from build123d import *

# Parameters (mm, degrees)
AUFSATZ_LINEAR_AUSTRAGEN1_DEPTH  = 13
AUFSATZ_LINEAR_START             = -13
SKIZZE2_W                        = 3
SKIZZE2_H                        = 12
AUFSATZ_LINEAR_AUSTRAGEN2_DEPTH  = 45
SKIZZE3_W                        = 8.8
SKIZZE3_H                        = 13
SKIZZE3_W_2                      = 18.8
AUFSATZ_LINEAR_AUSTRAGEN3_DEPTH  = 16.6
SKIZZE4_R                        = 1.7
SCHNITT_LINEAR_AUSTRAGEN1_DEPTH  = 4
SKIZZE6_R                        = 1.5
SCHNITT_LINEAR_AUSTRAGEN2_DEPTH  = 4
SCHNITT_LINEAR_START             = -3
SCHNITT_LINEAR_AUSTRAGEN4_DEPTH  = 2.5
SCHNITT_LINEAR_AUSTRAGEN6_DEPTH  = 91
SCHNITT_LINEAR_AUSTRAGEN7_REACH  = 2.5
SKIZZE11_R                       = 3.85
SCHNITT_LINEAR_START_2           = -15
SKIZZE12_W                       = 8
SKIZZE12_H                       = 5
SCHNITT_LINEAR_AUSTRAGEN8_DEPTH  = 16
SKIZZE13_W                       = 5
SKIZZE13_H                       = 8
SCHNITT_LINEAR_AUSTRAGEN9_DEPTH  = 91
SKIZZE14_R                       = 1
SCHNITT_LINEAR_AUSTRAGEN10_DEPTH = 71
AUFSATZ_LINEAR_START_2           = -3
SKIZZE15_R                       = 6
AUFSATZ_LINEAR_AUSTRAGEN4_DEPTH  = 4
SKIZZE16_R                       = 1.7
SCHNITT_LINEAR_AUSTRAGEN11_DEPTH = 3


with BuildPart() as part:
    # Skizze1 → Aufsatz-Linear austragen1 (new body)
    with BuildSketch(Plane.XY):
        Polygon((-45, 67), (-42, 67), (-42, 0), (42, 0), (42, 67), (45, 67), (45, -3), (-45, -3), align=None)
    extrude(amount=AUFSATZ_LINEAR_AUSTRAGEN1_DEPTH)

    # Skizze2 → Aufsatz-Linear austragen2 (add)
    with BuildSketch(Plane(origin=(0, 0, 0), x_dir=(-1, 0, 0), z_dir=(0, 0, -1)).offset(AUFSATZ_LINEAR_START)):
        with Locations((-43.5, 61)):
            Rectangle(SKIZZE2_W, SKIZZE2_H)
        with Locations((43.5, 61)):
            Rectangle(SKIZZE2_W, SKIZZE2_H)
    extrude(amount=AUFSATZ_LINEAR_AUSTRAGEN2_DEPTH)

    # Skizze3 → Aufsatz-Linear austragen3 (add)
    with BuildSketch(Plane(origin=(0, 0, 0), x_dir=(1, 0, 0), z_dir=(0, 1, 0))):
        with Locations((-37.6, -6.5)):
            Rectangle(SKIZZE3_W, SKIZZE3_H)
        with Locations((37.6, -6.5)):
            Rectangle(SKIZZE3_W, SKIZZE3_H)
        with Locations((0, -6.5)):
            Rectangle(SKIZZE3_W_2, SKIZZE3_H)
    extrude(amount=AUFSATZ_LINEAR_AUSTRAGEN3_DEPTH)

    # Skizze4 → Schnitt-Linear austragen1 (cut)
    with BuildSketch(Plane(origin=(0, 16.6, 0), x_dir=(1, 0, 0), z_dir=(0, 1, 0))):
        with Locations((-35.6, -6.5)):
            Circle(SKIZZE4_R)
        with Locations((-7, -6.5)):
            Circle(SKIZZE4_R)
        with Locations((7, -6.5)):
            Circle(SKIZZE4_R)
        with Locations((35.6, -6.5)):
            Circle(SKIZZE4_R)
    extrude(amount=-SCHNITT_LINEAR_AUSTRAGEN1_DEPTH, mode=Mode.SUBTRACT)

    # Skizze6 → Schnitt-Linear austragen2 (cut, through all)
    with BuildSketch(Plane.ZY.offset(-42)):
        with Locations((-26, 61)):
            Circle(SKIZZE6_R)
    extrude(amount=-SCHNITT_LINEAR_AUSTRAGEN2_DEPTH, mode=Mode.SUBTRACT)

    # Skizze7 → Schnitt-Linear austragen4 (cut)
    with BuildSketch(Plane.ZY.offset(45).offset(SCHNITT_LINEAR_START)):
        with BuildLine():
            Line((-25.802102804, 64.844910493), (-4.45864486, 63.746364638))
            ThreePointArc((-4.45864486, 63.746364638), (-1.85, 61), (-4.45864486, 58.253635362))
            Line((-4.45864486, 58.253635362), (-25.802102804, 57.155089507))
            ThreePointArc((-25.802102804, 57.155089507), (-29.85, 61), (-25.802102804, 64.844910493))
        make_face()
    extrude(amount=SCHNITT_LINEAR_AUSTRAGEN4_DEPTH, mode=Mode.SUBTRACT)

    # Skizze10 → Schnitt-Linear austragen6 (cut, through all)
    with BuildSketch(Plane.ZY.offset(45)):
        with BuildLine():
            Line((-26, 55), (-40.113250667, 55))
            Line((-40.113250667, 55), (-40.113250667, 67))
            Line((-40.113250667, 67), (-26, 67))
            ThreePointArc((-26, 67), (-32, 61), (-26, 55))
        make_face()
    extrude(amount=-SCHNITT_LINEAR_AUSTRAGEN6_DEPTH, mode=Mode.SUBTRACT)

    # Skizze11 → Schnitt-Linear austragen7 (cut, up to next)
    with BuildSketch(Plane(origin=(-44.5, 0, 0), x_dir=(0, 0, -1), z_dir=(1, 0, 0)), mode=Mode.PRIVATE) as schnitt_linear_austragen7_sk1:
        with Locations((26, 61)):
            Circle(SKIZZE11_R)
    schnitt_linear_austragen7_tool1 = extrude(schnitt_linear_austragen7_sk1.sketch, amount=-SCHNITT_LINEAR_AUSTRAGEN7_REACH, mode=Mode.PRIVATE) & part.part
    add(schnitt_linear_austragen7_tool1.solids().sort_by_distance((-44.5, 61, -26))[0], mode=Mode.SUBTRACT)

    # Skizze12 → Schnitt-Linear austragen8 (cut)
    with BuildSketch(Plane(origin=(45, 0, 0), x_dir=(0, 0, -1), z_dir=(1, 0, 0)).offset(SCHNITT_LINEAR_START_2)):
        with Locations((-4, 3.5)):
            Rectangle(SKIZZE12_W, SKIZZE12_H)
    schnitt_linear_austragen8 = extrude(amount=SCHNITT_LINEAR_AUSTRAGEN8_DEPTH, mode=Mode.SUBTRACT)

    # Spiegeln1: Schnitt-Linear austragen8 across plane
    add(schnitt_linear_austragen8.mirror(Plane.ZY), mode=Mode.SUBTRACT)

    # Skizze13 → Schnitt-Linear austragen9 (cut, through all)
    with BuildSketch(Plane.ZY.offset(45)):
        with Locations((6.5, 40.6)):
            Rectangle(SKIZZE13_W, SKIZZE13_H)
    extrude(amount=-SCHNITT_LINEAR_AUSTRAGEN9_DEPTH, mode=Mode.SUBTRACT)

    # Skizze14 → Schnitt-Linear austragen10 (cut, through all)
    with BuildSketch(Plane(origin=(0, -3, 0), x_dir=(-1, 0, 0), z_dir=(0, -1, 0))):
        with Locations((26.45, -6.15)):
            Circle(SKIZZE14_R)
        with Locations((-26.45, -6.15)):
            Circle(SKIZZE14_R)
    extrude(amount=-SCHNITT_LINEAR_AUSTRAGEN10_DEPTH, mode=Mode.SUBTRACT)

    # Skizze15 → Aufsatz-Linear austragen4 (add)
    with BuildSketch(Plane.ZY.offset(-42).offset(AUFSATZ_LINEAR_START_2)):
        with Locations((-26, 61)):
            Circle(SKIZZE15_R)
    extrude(amount=AUFSATZ_LINEAR_AUSTRAGEN4_DEPTH)

    # Skizze16 → Schnitt-Linear austragen11 (cut)
    with BuildSketch(Plane(origin=(45, 0, 0), x_dir=(0, 0, -1), z_dir=(1, 0, 0))):
        with Locations((26, 61)):
            Circle(SKIZZE16_R)
    extrude(amount=-SCHNITT_LINEAR_AUSTRAGEN11_DEPTH, mode=Mode.SUBTRACT)


solid = part.part
The listing builds one solid part. Answer for the finished solid, in the listing's coordinates (mm). A direction names the side the tool comes from. Coordinates: 2 decimals unless noted, no trailing zeros. Write each loop counter-clockwise with the first axis right and the second up, starting at its lowest first coordinate (ties: lowest second). Pieces come first, ordered by that corner, then holes. Notation, with made-up numbers: (-9.5, 78.5) - (-5.5, 78.5) arc R25 cw to (-5.5, 103.5) - close; hole circle Ø3 at (75.25, -17). An arc over 180 degrees is marked (long way). Put each result on its own line as item: value.
1. Determine the mould class of faces 4 (the face through (-9.4, 8, 7)), 5 (the face through (-43.48, 59.64, -29.6)), 6 (the face through (39, 3, 8)), 7 (the face through (43, 41, 9)) for opening direction Z: pulls with the +Z half, pulls with the -Z half, needs draft (parallel to the pull), parting line crosses it, or undercut.
Answer sheet:
face 4: needs draft
face 5: undercut
face 6: pulls with the -Z half
face 7: undercut
2. The part is cut by section A-A on y = 48.5. Give the vertices of the cut face in (x, z), plus the area to 3 significant figures.
Answer sheet:
outline: (-45, 0) - (-42, 0) - (-42, 13) - (-45, 13) - close; (42, 0) - (45, 0) - (45, 13) - (42, 13) - close
area: 78.0 mm^2
3. Flat-ended cylindrical pins translate along their axes: pin 1 Ø9.5 at (x, z) = (38, 4) entering from +Y; pin 2 Ø2.5 at (x, z) = (7, 7) entering from +Y; pin 3 Ø3 at (x, z) = (-7, 6.5) entering from +Y. Find the tip coordinate at first contact, or state that the pin passes through.
Answer sheet:
pin 1: stops at y = 67
pin 2: stops at y = 16.6
pin 3: stops at y = 12.6
4. A tool of negligible diameter and unlimited length cuts with its end or side. For faces 1 (the face through (-33.2, 8, 7)), 2 (the face through (-43, 55, -13)), 3 (the face through (-44, 41, 4)), from which of +Z, -Z, +X, -X, +Y, -Y can it reach the whole face along a straight path? Write none if from no direction.
Answer sheet:
face 1: +Z, -Z, +Y
face 2: -Z, +X, -X, -Y
face 3: +X, -X
5. The part is cut by section D-D on x = -7. Give the vertices of the cut face in (y, z).
Answer sheet:
outline: (-3, 0) - (16.6, 0) - (16.6, 4.8) - (12.6, 4.8) - (12.6, 8.2) - (16.6, 8.2) - (16.6, 13) - (-3, 13) - close
6. Find the intervals of material crossed by line 1 along X through (y, z) = (8, 1); line 2 along X through (y, z) = (-2.05, 6.15); line 3 along X through (y, z) = (23.5, 8.5), in increasing order. Write a range as from..to.
Answer sheet:
line 1: x = -45..-33.2, -9.4..9.4, 33.2..45
line 2: x = -45..-27.45, -25.45..25.45, 27.45..45
line 3: x = -45..-42, 42..45
7. The part is cut by section B-B on x = 26.45. Give the vertices of the cut face in (y, z).
Answer sheet:
outline: (-3, 0) - (0, 0) - (0, 5.15) - (-3, 5.15) - close; (-3, 7.15) - (0, 7.15) - (0, 13) - (-3, 13) - close
8. The part is cut by section C-C on x = -38.5. Give the vertices of the cut face in (y, z), plus the area to 3 significant figures.
Answer sheet:
outline: (-3, 0) - (1, 0) - (1, 8) - (6, 8) - (6, 0) - (16.6, 0) - (16.6, 13) - (-3, 13) - close
area: 215 mm^2
